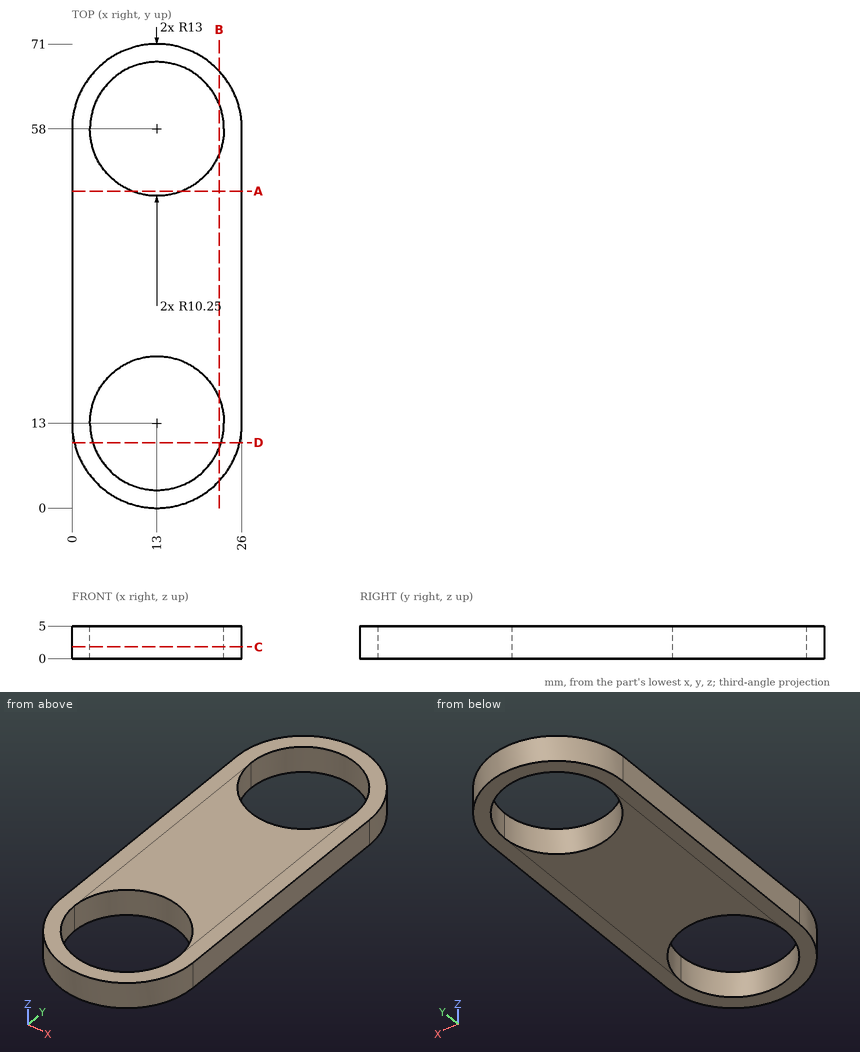
Part print with two shaded views. Sizes in mm from the minimum x, y, z corner. Coordinates: 2 decimals unless noted, no trailing zeros. Write each loop counter-clockwise with the first axis right and the second up, starting at its lowest first coordinate (ties: lowest second). Pieces come first, ordered by that corner, then holes.
1. Drop flat-ended pins along their axis: pin 1 (1.5 mm diameter, centred on x = 12, z = 3.5, fed in from -Y); pin 2 (1.5 mm diameter, centred on x = 2.5, z = 4.5, fed in from -Y). Give the stop position or say it passes through.
Answer block:
pin 1: stops at y = 0
pin 2: stops at y = 4.4
2. Band-saw the part on C-C, the plane z = 1.8. Give the cut face in (x, y).
Answer block:
outline: (0, 13) arc R13 ccw to (26, 13) - (26, 58) arc R13 ccw to (0, 58) - close; hole circle Ø20.5 at (13, 13); hole circle Ø20.5 at (13, 58)
3. Band-saw the part on A-A, the plane y = 48.5. Give the cut face in (x, z).
Answer block:
outline: (0, 0) - (9.15, 0) - (9.15, 5) - (0, 5) - close; (16.85, 0) - (26, 0) - (26, 5) - (16.85, 5) - close
4. Band-saw the part on B-B, the plane x = 22.5. Give the cut face in (y, z), and give its area (3 significant figures).
Answer block:
outline: (4.13, 0) - (9.15, 0) - (9.15, 5) - (4.13, 5) - close; (16.85, 0) - (54.15, 0) - (54.15, 5) - (16.85, 5) - close; (61.85, 0) - (66.87, 0) - (66.87, 5) - (61.85, 5) - close
area: 237 mm2
5. Band-saw the part on D-D, the plane y = 10. Give the cut face in (x, z), and give its area (3 significant figures).
Answer block:
outline: (0.35, 0) - (3.2, 0) - (3.2, 5) - (0.35, 5) - close; (22.8, 0) - (25.65, 0) - (25.65, 5) - (22.8, 5) - close
area: 28.5 mm2
6. Drill centre lines: probe 1 along Y at (x, z) = (7.5, 3); probe 2 along Y at (x, z) = (21.5, 0.9); probe 3 along X at (y, z) = (62, 3.7). Where is each one in solid material? Low to high.
Answer block:
probe 1: y = 1.22 to 4.35, 21.65 to 49.35, 66.65 to 69.78
probe 2: y = 3.16 to 7.27, 18.73 to 52.27, 63.73 to 67.84
probe 3: x = 0.63 to 3.56, 22.44 to 25.37
